For this review, take the finished solid that the model builds, in its own axes (mm). A direction names the side the tool comes from. Give positions to 0.01 mm unless a question says otherwise; leave off trailing zeros. Loops run counter-clockwise (first coordinate to the right, second up) from the corner with the lowest first, then second, coordinate; pieces in that order, holes last.
```python
from build123d import *

# Parameters (mm, degrees)
SKETCH1_R           = 1.5
BOSS_EXTRUDE1_DEPTH = 0.8


with BuildPart() as part:
    # Sketch1 → Boss-Extrude1 (new, symmetric)
    # profile 1 of 9: a face of its own
    with BuildSketch(Plane(origin=(0, 0, 0), x_dir=(1, 0, 0), z_dir=(0, 1, 0))):
        with BuildLine():
            ThreePointArc((-19.05, -4.699), (-16.002, -7.747), (-19.05, -10.795))
            Line((-19.05, -10.795), (19.05, -10.795))
            ThreePointArc((19.05, -10.795), (16.002, -7.747), (19.05, -4.699))
            Line((19.05, -4.699), (19.05, 4.699))
            ThreePointArc((19.05, 4.699), (16.002, 7.747), (19.05, 10.795))
            Line((19.05, 10.795), (-19.05, 10.795))
            ThreePointArc((-19.05, 10.795), (-16.002, 7.747), (-19.05, 4.699))
            Line((-19.05, 4.699), (-19.05, -4.699))
        make_face()
    # profile 2 of 9: a face of its own
    with BuildSketch(Plane(origin=(0, 0, 0), x_dir=(1, 0, 0), z_dir=(0, 1, 0))):
        with BuildLine():
            Line((-22.075, -10.795), (-19.05, -10.795))
            Line((-19.05, -10.795), (-19.05, -4.699))
            Line((-19.05, -4.699), (-22.075, -4.699))
            ThreePointArc((-22.075, -4.699), (-25.123, -7.747), (-22.075, -10.795))
        make_face()
        with Locations(Location((-22.075, -7.747, 0), (0, 0, 270))):
            Circle(SKETCH1_R, mode=Mode.SUBTRACT)
    # profile 3 of 9: a face of its own
    with BuildSketch(Plane(origin=(0, 0, 0), x_dir=(1, 0, 0), z_dir=(0, 1, 0))):
        with BuildLine():
            Line((-19.05, -4.699), (-19.05, -10.795))
            ThreePointArc((-19.05, -10.795), (-16.002, -7.747), (-19.05, -4.699))
        make_face()
    # profile 4 of 9: a face of its own
    with BuildSketch(Plane(origin=(0, 0, 0), x_dir=(1, 0, 0), z_dir=(0, 1, 0))):
        with BuildLine():
            Line((-19.05, 10.795), (-19.05, 4.699))
            ThreePointArc((-19.05, 4.699), (-16.002, 7.747), (-19.05, 10.795))
        make_face()
    # profile 5 of 9: a face of its own
    with BuildSketch(Plane(origin=(0, 0, 0), x_dir=(1, 0, 0), z_dir=(0, 1, 0))):
        with BuildLine():
            Line((-22.075, 4.699), (-19.05, 4.699))
            Line((-19.05, 4.699), (-19.05, 10.795))
            Line((-19.05, 10.795), (-22.075, 10.795))
            ThreePointArc((-22.075, 10.795), (-25.123, 7.747), (-22.075, 4.699))
        make_face()
        with Locations(Location((-22.075, 7.747, 0), (0, 0, 270))):
            Circle(SKETCH1_R, mode=Mode.SUBTRACT)
    # profile 6 of 9: a face of its own
    with BuildSketch(Plane(origin=(0, 0, 0), x_dir=(1, 0, 0), z_dir=(0, 1, 0))):
        with BuildLine():
            ThreePointArc((19.05, 10.795), (16.002, 7.747), (19.05, 4.699))
            Line((19.05, 4.699), (19.05, 10.795))
        make_face()
    # profile 7 of 9: a face of its own
    with BuildSketch(Plane(origin=(0, 0, 0), x_dir=(1, 0, 0), z_dir=(0, 1, 0))):
        with BuildLine():
            Line((19.05, 10.795), (19.05, 4.699))
            Line((19.05, 4.699), (22.075, 4.699))
            ThreePointArc((22.075, 4.699), (25.123, 7.747), (22.075, 10.795))
            Line((22.075, 10.795), (19.05, 10.795))
        make_face()
        with Locations(Location((22.075, 7.747, 0), (0, 0, 270))):
            Circle(SKETCH1_R, mode=Mode.SUBTRACT)
    # profile 8 of 9: a face of its own
    with BuildSketch(Plane(origin=(0, 0, 0), x_dir=(1, 0, 0), z_dir=(0, 1, 0))):
        with BuildLine():
            Line((19.05, -4.699), (19.05, -10.795))
            Line((19.05, -10.795), (22.075, -10.795))
            ThreePointArc((22.075, -10.795), (25.123, -7.747), (22.075, -4.699))
            Line((22.075, -4.699), (19.05, -4.699))
        make_face()
        with Locations(Location((22.075, -7.747, 0), (0, 0, 270))):
            Circle(SKETCH1_R, mode=Mode.SUBTRACT)
    # profile 9 of 9: a face of its own
    with BuildSketch(Plane(origin=(0, 0, 0), x_dir=(1, 0, 0), z_dir=(0, 1, 0))):
        with BuildLine():
            ThreePointArc((19.05, -4.699), (16.002, -7.747), (19.05, -10.795))
            Line((19.05, -10.795), (19.05, -4.699))
        make_face()
    extrude(amount=BOSS_EXTRUDE1_DEPTH, both=True)


solid = part.part
```
Item 1: For L1, parallel to Z at x = 22, y = 0.35 (3 decimals); L2, parallel to X at y = -0.7, z = 2.5, list the stretches that pass through material, from the lowest coordinate up.
Answer:
L1: z = -10.795 to -9.245, -6.249 to -4.699, 4.699 to 6.249, 9.245 to 10.795
L2: x = -19.05 to 19.05
Item 2: Take a section at A-A on y = 0.35. Give the boundary of the cut face in (x, z) (3 decimals).
Answer:
outline: (-22.075, -10.795) - (22.075, -10.795) arc R3.048 ccw to (22.075, -4.699) - (19.05, -4.699) - (19.05, 4.699) - (22.075, 4.699) arc R3.048 ccw to (22.075, 10.795) - (-22.075, 10.795) arc R3.048 ccw to (-22.075, 4.699) - (-19.05, 4.699) - (-19.05, -4.699) - (-22.075, -4.699) arc R3.048 ccw to start; hole circle Ø3 at (-22.075, -7.747); hole circle Ø3 at (-22.075, 7.747); hole circle Ø3 at (22.075, -7.747); hole circle Ø3 at (22.075, 7.747)
Item 3: Tool access review of faces 5 (the flat face through (-19.05, 0, 0)), 6 (the flat face through (0, 0, -10.795)), 7 (the flat face through (19.05, 0, 0)): name each direction out of +Z, -Z, +X, -X, +Y, -Y from which nothing blocks a thin tool from reaching the whole face with its end or side.
Answer:
face 5: -X, +Y, -Y
face 6: -Z, +X, -X, +Y, -Y
face 7: +X, +Y, -Y
Item 4: Clearance check with a flat-ended pin moving along its axis: pin 1 Ø2.5 at (x, z) = (-22.075, -7.747) entering from +Y. State where the tip first meets the part, or that it passes through.
Answer:
pin 1: passes through
Item 5: Take a section at B-B on z = -2.25. Give the boundary of the cut face in (x, y), and give its area (3 significant figures).
Answer:
outline: (-19.05, -0.8) - (19.05, -0.8) - (19.05, 0.8) - (-19.05, 0.8) - close
area: 61.0 mm2
Item 6: The part is to be moulded in two halves that separate along Z. For faces 1 (the flat face through (0, 0, 10.795)), 2 (the cylindrical face through (25.122, 0.011, 7.814)), 3 (the flat face through (0, -0.8, 0)), 4 (the flat face through (21, 0, 4.699)), say which applies: released by +Z, released by -Z, zero draft, split by the parting line, or undercut.
Answer:
face 1: released by +Z
face 2: undercut
face 3: zero draft
face 4: undercut
